Geometry: final body of the model. Coordinates: model frame, mm. A direction names the side the tool comes from. Give positions to 0.01 mm unless a question says otherwise; leave off trailing zeros. Write each loop counter-clockwise with the first axis right and the second up, starting at its lowest first coordinate (ties: lowest second). Pieces come first, ordered by that corner, then holes.
Q1. Draft query along X for faces 6 (the face through (-13, 80, -7)), 7 (the face through (-14, 86, -10)), 8 (the face through (24.71, 18.675, -20.185)), 9 (the face through (-13, 6, 12)). Return one class per face: pulls with the +X half, pulls with the -X half, needs draft (parallel to the pull), parting line crosses it, or undercut.
Q2. Cut plane C-C on x = -9.5. Return the cut outline in (y, z).
Q3. Cut plane D-D on y = 8. Return the cut outline in (x, z), plus the area to 3 significant figures.
Q4. Cut plane A-A on y = 38.5. Return the cut outline in (x, z), plus the area to 3 significant figures.
Q5. Pin query (flat end, axial travel): pin 1 (16 mm diameter, centred on x = -56, y = 15.5, fed in from +Z); pin 2 (9.5 mm diameter, centred on x = 21.85, z = -4.79, fed in from -Y); pin 3 (11.5 mm diameter, centred on x = 18, z = 15, fed in from +Y); pin 4 (11 mm diameter, centred on y = 45, z = -7, fed in from -X). Return the tip coordinate at first contact, or that it passes through.
Q6. Cut plane B-B on z = 16.5. Return the cut outline in (x, y).
Q7. Line query: L1, parallel to X at y = 72, z = -21; L2, parallel to Z at x = -2, y = 76.5; L3, parallel to X at y = 58.5, z = -36. Output: solid intervals per line, ascending.
Q8. Reachability of faces 1 (the face through (-7.15, 46, -7)), 2 (the face through (-47, 13, -12.79)), 3 (the face through (-22, 45, -28.79)), 4 (the face through (-47, 13, -27.79)), 5 (the face through (5.44, 21.31, 12.41)) from +Z, -Z, +X, -X, +Y, -Y: full face, straight path, thin tool, end or side. Return the list, or none.
```python
from build123d import *

# Parameters (mm, degrees)
SKETCH_1_W          = 96
SKETCH_1_H          = 70
SKETCH_1_R          = 3
EXTRUDE_1_DEPTH     = 6
SKETCH_2_W          = 56
SKETCH_2_H          = 37
SKETCH_2_W_2        = 40
SKETCH_2_H_2        = 17
EXTRUDE_2_DEPTH     = 80
EXTRUDE_3_DEPTH     = 7.5
EXTRUDE_4_DEPTH     = 25
CUT_EXTRUDE_1_DEPTH = 124.93663618
SKETCH_10_W         = 24
SKETCH_10_H         = 30.908347595
CUT_EXTRUDE_2_DEPTH = 80
FILLET_1_R          = 2


with BuildPart() as part:
    # 草图1 → 凸台-拉伸1 (new body)
    with BuildSketch(Plane(origin=(0, 0, 0), x_dir=(1, 0, 0), z_dir=(0, 1, 0))):
        with Locations((-13.149732523, 8.78973091)):
            Rectangle(SKETCH_1_W, SKETCH_1_H)
        with Locations(Location((21.850267477, 4.78973091, 0), (0, 0, 270))):
            Circle(SKETCH_1_R, mode=Mode.SUBTRACT)
        with Locations(Location((-48.149732523, 4.78973091, 0), (0, 0, 270))):
            Circle(SKETCH_1_R, mode=Mode.SUBTRACT)
        with Locations(Location((21.850267477, -15.21026909, 0), (0, 0, 270))):
            Circle(SKETCH_1_R, mode=Mode.SUBTRACT)
        with Locations(Location((-48.149732523, -15.21026909, 0), (0, 0, 270))):
            Circle(SKETCH_1_R, mode=Mode.SUBTRACT)
        with Locations(Location((21.850267477, 34.78973091, 0), (0, 0, 270))):
            Circle(SKETCH_1_R, mode=Mode.SUBTRACT)
        with Locations(Location((-48.149732523, 34.78973091, 0), (0, 0, 270))):
            Circle(SKETCH_1_R, mode=Mode.SUBTRACT)
    extrude(amount=EXTRUDE_1_DEPTH)

    # 草图2 → 凸台-拉伸2 (add)
    with BuildSketch(Plane(origin=(0, 6, 0), x_dir=(1, 0, 0), z_dir=(0, 1, 0))):
        with Locations((-13.149732523, 20.28973091)):
            Rectangle(SKETCH_2_W, SKETCH_2_H)
        with Locations((-13.149732523, 20.28973091)):
            Rectangle(SKETCH_2_W_2, SKETCH_2_H_2, mode=Mode.SUBTRACT)
    extrude(amount=EXTRUDE_2_DEPTH)

    # 草图5 → 凸台-拉伸3 (add, symmetric)
    with BuildSketch(Plane.XY.offset(-20.28973091)):
        Polygon((-61.149732523, 6), (-41.149732523, 31), (-41.149732523, 6), align=None)
        Polygon((14.850267477, 31), (34.850267477, 6), (14.850267477, 6), align=None)
    extrude(amount=EXTRUDE_3_DEPTH, both=True)

    # 草图8 → 凸台-拉伸4 (add, symmetric)
    with BuildSketch(Plane(origin=(-13.149732523, 0, 0), x_dir=(0, 0, -1), z_dir=(1, 0, 0))):
        Polygon((-26.21026909, 6), (1.78973091, 37.060621439), (1.78973091, 6), align=None)
    extrude(amount=EXTRUDE_4_DEPTH, both=True)

    # 草图9 → 切除-拉伸1 (cut, through all)
    with BuildSketch(Plane(origin=(0, 0, -38.78973091), x_dir=(-1, 0, 0), z_dir=(0, 0, -1))):
        with BuildLine():
            Line((19.149732523, 74), (19.149732523, 18))
            ThreePointArc((19.149732523, 18), (13.149732523, 12), (7.149732523, 18))
            Line((7.149732523, 18), (7.149732523, 74))
            ThreePointArc((7.149732523, 74), (13.149732523, 80), (19.149732523, 74))
        make_face()
    extrude(amount=-CUT_EXTRUDE_1_DEPTH, mode=Mode.SUBTRACT)

    # 草图10 → 切除-拉伸2 (cut)
    with BuildSketch(Plane(origin=(0, 86, 0), x_dir=(1, 0, 0), z_dir=(0, 1, 0))):
        with Locations((-13.149732523, -13.664442888)):
            Rectangle(SKETCH_10_W, SKETCH_10_H)
    extrude(amount=-CUT_EXTRUDE_2_DEPTH, mode=Mode.SUBTRACT)

    # 圆角1
    fillet_1_edges = [part.edges().sort_by_distance(p)[0] for p in [
        (14.850267477, 86, -20.28973091),
        (-13.149732523, 86, -38.78973091),
        (-41.149732523, 86, -20.28973091),
        (-13.149732523, 86, -1.78973091),
    ]]
    fillet(fillet_1_edges, radius=FILLET_1_R)


solid = part.part
```
Data:
1. face 6: undercut
1. face 7: needs draft
1. face 8: pulls with the +X half
1. face 9: undercut
2. outline: (0, -43.79) - (6, -43.79) - (6, -38.79) - (13.24, -38.79) - (13.24, -28.79) - (6, -28.79) - (6, -11.79) - (13.24, -11.79) - (13.24, -1.79) - (6, -1.79) - (6, 26.21) - (0, 26.21) - close; (78.76, -38.79) - (84, -38.79) arc R2 ccw to (86, -36.79) - (86, -28.79) - (78.76, -28.79) - close; (78.76, -11.79) - (86, -11.79) - (86, -3.79) arc R2 ccw to (84, -1.79) - (78.76, -1.79) - close
3. outline: (-59.55, -27.79) - (-41.15, -27.79) - (-41.15, -38.79) - (14.85, -38.79) - (14.85, -27.79) - (33.25, -27.79) - (33.25, -12.79) - (14.85, -12.79) - (14.85, -1.79) - (11.85, -1.79) - (11.85, 24.41) - (-1.15, 24.41) - (-1.15, -1.79) - (-25.15, -1.79) - (-25.15, 24.41) - (-38.15, 24.41) - (-38.15, -1.79) - (-41.15, -1.79) - (-41.15, -12.79) - (-59.55, -12.79) - close; hole (-33.15, -28.79) - (6.85, -28.79) - (6.85, -11.79) - (-33.15, -11.79) - close
3. area: 2,630 mm2
4. outline: (-41.15, -38.79) - (-19.15, -38.79) - (-19.15, -28.79) - (-33.15, -28.79) - (-33.15, -11.79) - (-19.15, -11.79) - (-19.15, -1.79) - (-41.15, -1.79) - close; (-7.15, -38.79) - (14.85, -38.79) - (14.85, -1.79) - (-7.15, -1.79) - (-7.15, -11.79) - (6.85, -11.79) - (6.85, -28.79) - (-7.15, -28.79) - close
4. area: 1,150 mm2
5. pin 1: stops at z = -12.79
5. pin 2: stops at y = 0
5. pin 3: stops at y = 6
5. pin 4: stops at x = -41.15
6. outline: (-61.15, 0) - (-50.86, 0) - (-50.86, 6) - (-61.15, 6) - close; (-45.44, 0) - (19.14, 0) - (19.14, 6) - (11.85, 6) - (11.85, 16.77) - (-1.15, 16.77) - (-1.15, 6) - (-25.15, 6) - (-25.15, 16.77) - (-38.15, 16.77) - (-38.15, 6) - (-45.44, 6) - close; (24.56, 0) - (34.85, 0) - (34.85, 6) - (24.56, 6) - close
7. L1: x = -41.15 to -33.15, 6.85 to 14.85
7. L2: z = -38.79 to -28.79, -11.79 to -1.79
7. L3: x = -41.15 to -19.15, -7.15 to 14.85
8. face 1: +Z, -Z
8. face 2: +Z, -X, +Y
8. face 3: +Y
8. face 4: -Z, -X, +Y
8. face 5: +Z, +X, -X, +Y
